from build123d import *

# Parameters (mm, degrees)
BOSS_EXTRUDE1_DEPTH = 7
BOSS_EXTRUDE2_START = 1
BOSS_EXTRUDE2_DEPTH = 1
SKETCH3_R           = 1.75
CUT_EXTRUDE1_DEPTH  = 29.268910739


with BuildPart() as part:
    # Sketch1 → Boss-Extrude1 (new body)
    with BuildSketch(Plane.XZ.offset(-0.5)):
        with BuildLine():
            Line((-18.277494739, -8.221105303), (-20.043904797, -12.822760829))
            ThreePointArc((-20.043904797, -12.822760829), (-19.457528855, -16.326805286), (-16.10854182, -17.512743794))
            Line((-16.10854182, -17.512743794), (-11.270061894, -16.57223857))
            ThreePointArc((-11.270061894, -16.57223857), (-8.617981259, -16.416224916), (-6.018410533, -16.964042403))
            ThreePointArc((-6.018410533, -16.964042403), (11.570176974, -13.788799976), (17.751406503, 2.981202305))
            ThreePointArc((17.751406503, 2.981202305), (17.663322313, 5.636407218), (18.277494739, 8.221105303))
            Line((18.277494739, 8.221105303), (20.043904797, 12.822760829))
            ThreePointArc((20.043904797, 12.822760829), (19.457528855, 16.326805286), (16.10854182, 17.512743794))
            Line((16.10854182, 17.512743794), (11.270061894, 16.57223857))
            ThreePointArc((11.270061894, 16.57223857), (8.617981259, 16.416224916), (6.018410533, 16.964042403))
            ThreePointArc((6.018410533, 16.964042403), (-11.570176974, 13.788799976), (-17.751406503, -2.981202305))
            ThreePointArc((-17.751406503, -2.981202305), (-17.663322313, -5.636407218), (-18.277494739, -8.221105303))
        make_face()
    extrude(amount=-BOSS_EXTRUDE1_DEPTH)

    # Sketch2 → Boss-Extrude2 (add)
    with BuildSketch(Plane.XZ.offset(-0.5).offset(BOSS_EXTRUDE2_START)):
        with BuildLine():
            Line((-7.793099068, -15.677037579), (-7.400434194, -15.347552628))
            ThreePointArc((-7.400434194, -15.347552628), (-7.14763906, -15.235302983), (-6.873851261, -15.274617153))
            ThreePointArc((-6.873851261, -15.274617153), (10.766716645, -12.831273242), (16.236193142, 4.117012581))
            ThreePointArc((16.236193142, 4.117012581), (16.245018994, 4.393467763), (16.39946073, 4.622930425))
            Line((16.39946073, 4.622930425), (16.792125603, 4.952415375))
            ThreePointArc((16.792125603, 4.952415375), (17.323359362, 5.02322924), (17.613508913, 4.572632804))
            ThreePointArc((17.613508913, 4.572632804), (17.650630104, 3.77415969), (17.751406503, 2.981202305))
            ThreePointArc((17.751406503, 2.981202305), (11.570176974, -13.788799976), (-6.018410533, -16.964042403))
            ThreePointArc((-6.018410533, -16.964042403), (-6.781821476, -16.72710142), (-7.561717962, -16.551890782))
            ThreePointArc((-7.561717962, -16.551890782), (-7.955084885, -16.187904005), (-7.793099068, -15.677037579))
        make_face()
        with BuildLine():
            Line((7.793099068, 15.677037579), (7.400434194, 15.347552628))
            ThreePointArc((7.400434194, 15.347552628), (7.14763906, 15.235302983), (6.873851261, 15.274617153))
            ThreePointArc((6.873851261, 15.274617153), (-10.766716645, 12.831273242), (-16.236193142, -4.117012581))
            ThreePointArc((-16.236193142, -4.117012581), (-16.245018994, -4.393467763), (-16.39946073, -4.622930425))
            Line((-16.39946073, -4.622930425), (-16.792125603, -4.952415375))
            ThreePointArc((-16.792125603, -4.952415375), (-17.323359362, -5.02322924), (-17.613508913, -4.572632804))
            ThreePointArc((-17.613508913, -4.572632804), (-17.650630104, -3.77415969), (-17.751406503, -2.981202305))
            ThreePointArc((-17.751406503, -2.981202305), (-11.570176974, 13.788799976), (6.018410533, 16.964042403))
            ThreePointArc((6.018410533, 16.964042403), (6.781821476, 16.72710142), (7.561717962, 16.551890782))
            ThreePointArc((7.561717962, 16.551890782), (7.955084885, 16.187904005), (7.793099068, 15.677037579))
        make_face()
    extrude(amount=-BOSS_EXTRUDE2_DEPTH)

    # Sketch3 → Cut-Extrude1 (cut, through all)
    with BuildSketch(Plane(origin=(0, 7.5, 0), x_dir=(-1, 0, 0), z_dir=(0, 1, 0))):
        with Locations(Location((-16.776373304, 14.077048652, 0), (0, 0, 90))):
            Circle(SKETCH3_R)
        with Locations(Location((16.776373304, -14.077048652, 0), (0, 0, 90))):
            Circle(SKETCH3_R)
    extrude(amount=-CUT_EXTRUDE1_DEPTH, mode=Mode.SUBTRACT)


solid = part.part
The model under review builds one solid part; all positions refer to its coordinate system, in mm. A direction names the side the tool comes from. Coordinates: 2 decimals unless noted, no trailing zeros. Write each loop counter-clockwise with the first axis right and the second up, starting at its lowest first coordinate (ties: lowest second). Pieces come first, ordered by that corner, then holes. Notation, with made-up numbers: M -18,44.5 L 2,44.5 A11 ccw 2,49.5 Z; hole C -9.5,-37 d7. An arc over 180 degrees is marked long. Put each result on its own line as item: value.
1) Draft analysis for pull direction Z (two halves, no side actions). For faces 1 (the cylindrical face through (-18.485, 4.049, -14.456)), 2 (the flat face through (-11, -0.5, 13)), 3 (the flat face through (-19.15, 3.95, -10.49)), state which applies: released by +Z, released by -Z, zero draft, split by the parting line, or undercut.
Computed:
face 1: undercut
face 2: zero draft
face 3: released by +Z
2) Add section B-B on z = -14. Give the boundary of the cut face in (x, y).
Computed:
outline: M -20.28,0.5 L -18.52,0.5 L -18.52,7.5 L -20.28,7.5 Z; M -15.03,0.5 L 9.2,0.5 L 9.2,-0.5 L 11.31,-0.5 L 11.31,7.5 L -15.03,7.5 Z
3) Add section A-A on y = 0. Give the boundary of the cut face in (x, z), then the cut area to 3 significant figures.
Computed:
outline: M -17.75,-2.98 A10 cw -17.61,-4.57 A0.5 ccw -16.79,-4.95 L -16.4,-4.62 A0.5 ccw -16.24,-4.12 A16.75 cw 6.87,15.27 A0.5 ccw 7.4,15.35 L 7.79,15.68 A0.5 ccw 7.56,16.55 A10 cw 6.02,16.96 A18 ccw Z; M -7.79,-15.68 A0.5 ccw -7.56,-16.55 A10 cw -6.02,-16.96 A18 ccw 17.75,2.98 A10 cw 17.61,4.57 A0.5 ccw 16.79,4.95 L 16.4,4.62 A0.5 ccw 16.24,4.12 A16.75 cw -6.87,-15.27 A0.5 ccw -7.4,-15.35 Z
area: 101 mm2
4) Wall thickness on probe 1 along Y at (x, z) = (-0.5, 8); probe 2 along X at (y, z) = (3.75, -0.5); probe 3 along X at (y, z) = (2.25, -15): over which ranges is each line inside the solid? List them lowest first. Write a range as [from, to].
Computed:
probe 1: y = [0.5, 7.5]
probe 2: x = [-17.99, 17.99]
probe 3: x = [-20.15, -18.26], [-15.29, 9.95]
5) For faces 4 (the cylindrical face through (10.56, -0.01, -13)), 5 (the cylindrical face through (7.95, -0.01, 16.2)), 6 (the flat face through (13.72, 3.95, 17.05)), 7 (the cylindrical face through (-7.95, -0.01, -16.2)), 8 (the flat face through (-13.72, 3.95, -17.05)), list the 3-axis set-ups (+Z, -Z, +X, -X, +Y, -Y) from which the entire face can be reached by the end or side of a thin tool; tool diameter is ignored.
Computed:
face 4: -Y
face 5: +X, -Y
face 6: +Z, +Y, -Y
face 7: -X, -Y
face 8: -Z, +Y, -Y
6) Clearance check with flat-ended pins moving along their axes: pin 1 Ø4 at (x, z) = (13, -0.5) entering from -Y; pin 2 Ø3 at (y, z) = (1, -11) entering from -X. State where each tip first meets the part, or that it passes through.
Computed:
pin 1: stops at y = 0.5
pin 2: stops at x = -19.92
7) Add section D-D on z = -1.5. Give the boundary of the cut face in (x, y).
Computed:
outline: M -17.94,-0.5 L -16.68,-0.5 L -16.68,0.5 L 16.68,0.5 L 16.68,-0.5 L 17.94,-0.5 L 17.94,7.5 L -17.94,7.5 Z
8) Add section C-C on x = 2.5. Give the boundary of the cut face in (y, z), then the cut area to 3 significant figures.
Computed:
outline: M -0.5,-17.83 L 7.5,-17.83 L 7.5,17.83 L -0.5,17.83 L -0.5,16.56 L 0.5,16.56 L 0.5,-16.56 L -0.5,-16.56 Z
area: 252 mm2
